Check sheet for the modelled part. Datum: model origin and axes. Units: mm. Face numbers are marked on the shaded views. A direction names the side the tool comes from. Coordinates: 2 decimals unless noted, no trailing zeros. Loops run counter-clockwise (first coordinate to the right, second up) from the corner with the lowest first, then second, coordinate; pieces in that order, holes last.
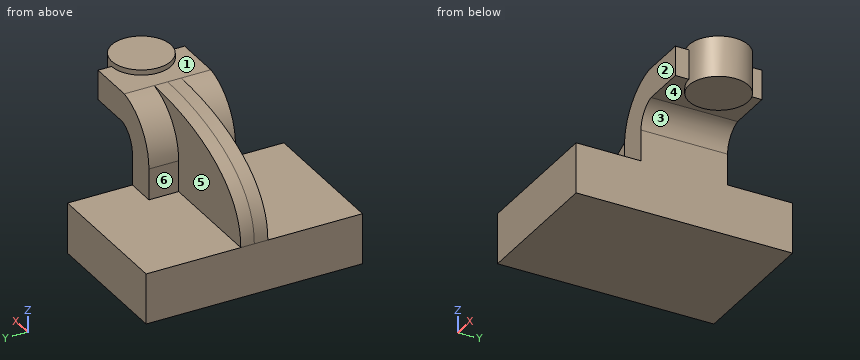
```python
from build123d import *

# Parameters (mm, degrees)
F1_DEPTH = 63.5
F0_W     = 17.417691648
F0_H     = 17.4204483628
F2_DEPTH = 25.4
F3_DEPTH = 7.9375


with BuildPart() as f1:
    # F0 (on Front) → F1 (new body, symmetric)
    with BuildSketch(Plane.XZ):
        Polygon((-24.308366701, 9.6553536132), (-24.308366701, -20.018171519), (58.7199889123, -20.018171519), (58.7199889123, 9.6553536132), (41.2995405495, 9.6553536132), align=None)
    extrude(amount=F1_DEPTH, both=True)

    # F0 (on Front) → F2 (join, symmetric)
    with BuildSketch(Plane.XZ):
        with BuildLine():
            Line((41.2995405495, 9.6553536132), (58.7199889123, 9.6553536132))
            Line((58.7199889123, 9.6553536132), (58.7199889123, 27.9359869646))
            ThreePointArc((58.7199889123, 27.9359869646), (61.6462339418, 36.6784025907), (69.2457072501, 41.8976694345))
            Line((69.2457072501, 41.8976694345), (77.5875747204, 41.8976694345))
            Line((77.5875747204, 41.8976694345), (77.5875747204, 59.3181177974))
            Line((77.5875747204, 59.3181177974), (67.2831763104, 59.3181177974))
            ThreePointArc((67.2831763104, 59.3181177974), (48.6385264432, 48.3074588245), (41.2995405495, 27.9359869646))
            Line((41.2995405495, 27.9359869646), (41.2995405495, 9.6553536132))
        make_face()
        with Locations((86.2964205444, 50.607893616)):
            Rectangle(F0_W, F0_H)
    extrude(amount=F2_DEPTH, both=True)

    # F0 (on Front) → F3 (join, symmetric)
    with BuildSketch(Plane.XZ):
        with BuildLine():
            add(Edge.make_bspline(
                [(-24.308366701, 9.6553536132), (-24.308366701, 46.6815978289), (26.0343328118, 59.3484714627), (67.2831763104, 59.3181177974)],
                knots=[0, 0, 0, 0, 104.1892551928, 104.1892551928, 104.1892551928, 104.1892551928], degree=3))
            Line((-24.308366701, 9.6553536132), (41.2995405495, 9.6553536132))
            Line((41.2995405495, 9.6553536132), (41.2995405495, 27.9359869646))
            ThreePointArc((41.2995405495, 27.9359869646), (48.6385264432, 48.3074588245), (67.2831763104, 59.3181177974))
        make_face()
    extrude(amount=F3_DEPTH, both=True)

    # F0 (on Front) → F4 (revolve)
    with BuildSketch(Plane.XZ):
        Polygon((95.0052663684, 62.3890832067), (95.0052663684, 59.3181177974), (95.0052663684, 41.8976694345), (95.0052663684, 38.4824350476), (112.4229580164, 38.4824350476), (112.4229580164, 62.3890832067), align=None)
    revolve(axis=Axis((95.0052663684, 0, 50.4357591271), (0, 0, 1)))


solid = f1.part
```
1) Section check B-B on x = 85. Enter the section's corners in (y, z).
Answer sheet:
outline: (-25.4, 41.9) - (-14.26, 41.9) - (-14.26, 38.48) - (14.26, 38.48) - (14.26, 41.9) - (25.4, 41.9) - (25.4, 59.32) - (14.26, 59.32) - (14.26, 62.39) - (-14.26, 62.39) - (-14.26, 59.32) - (-25.4, 59.32) - close
2) Mould release check, pull along X, two halves, no side actions. Record for the marked faces 4, 5 and 6: +X half, -X half, draft (parallel to the pull), parting line (faces both ways), or undercut.
Answer sheet:
face 4: undercut
face 5: draft
face 6: -X half
3) Scan lines: line 1 (Z direction, x = -6, y = 17); line 2 (Y direction, x = 40.5, z = 53); line 3 (X direction, y = 22.5, z = 6.5). Record each from-to range of solid material in increasing order.
Answer sheet:
line 1: z = -20.02 to 9.66
line 2: y = -7.94 to 7.94
line 3: x = -24.31 to 58.72
4) Depth check by flat-ended pin: pin 1 (12 mm diameter, centred on x = 61.5, z = 44.5, fed in from -Y); pin 2 (4 mm diameter, centred on x = 50, y = 7.5, fed in from +Z); pin 3 (9 mm diameter, centred on y = -22.5, z = 47, fed in from +X); pin 4 (19 mm diameter, centred on y = -18, z = 15, fed in from -X). Enter the tip coordinate at first touch or a pass-through.
Answer sheet:
pin 1: stops at y = -25.4
pin 2: stops at z = 58.75
pin 3: stops at x = 95.01
pin 4: stops at x = -24.31
5) Section check C-C on z = -1. Enter the section's corners in (x, y).
Answer sheet:
outline: (-24.31, -63.5) - (58.72, -63.5) - (58.72, 63.5) - (-24.31, 63.5) - close
6) Section check A-A on y = -15. Enter the section's corners in (x, z).
Answer sheet:
outline: (-24.31, -20.02) - (58.72, -20.02) - (58.72, 27.94) arc R14.52 cw to (69.25, 41.9) - (86.15, 41.9) - (86.15, 38.48) - (103.86, 38.48) - (103.86, 62.39) - (86.15, 62.39) - (86.15, 59.32) - (67.28, 59.32) arc R31.94 ccw to (41.3, 27.94) - (41.3, 9.66) - (-24.31, 9.66) - close
7) Section check D-D on y = -34.5. Enter the section's corners in (x, z), plus the area to 3 significant figures.
Answer sheet:
outline: (-24.31, -20.02) - (58.72, -20.02) - (58.72, 9.66) - (-24.31, 9.66) - close
area: 2,460 mm2
8) Set-up check for the marked faces 1, 2 and 3: record each of +Z, -Z, +X, -X, +Y, -Y from which the full face is reachable in a straight line by a thin tool's end or side.
Answer sheet:
face 1: +Z, -X
face 2: +Z, +X, -X, -Y
face 3: -Z, +Y, -Y
